Build history of the part. All positions in model axes, mm. A direction names the side the tool comes from. Give positions to 0.01 mm unless a question says otherwise; leave off trailing zeros. Loops run counter-clockwise (first coordinate to the right, second up) from the corner with the lowest first, then second, coordinate; pieces in that order, holes last. Notation, with made-up numbers: M 41.25,89.25 L 74.25,89.25 A16 ccw 74.25,106.25 Z; hole C 88.25,-24 d10. An arc over 180 degrees is marked long. Answer as a JSON object with one key per item and string values. Group by question number.
1. Slice it at C-C (z = -5). Give the number of separate pieces and of enclosed holes in the cut face, then the cut area to 3 significant figures.
2. Mould opens along Y. For faces 4 (the face through (9.203, 21.327, -2.555)), 5 (the face through (-0.03, 24.43, -56.15)), 6 (the face through (-6, 12, -2)) say: released by +Y, released by -Y, zero draft, split by the parting line, or undercut.
3. Drop flat-ended pins along their axis: pin 1 Ø5.5 at (x, z) = (0, -26.75) entering from +Y; pin 2 Ø6 at (y, z) = (3, -9.5) entering from +X; pin 3 Ø4 at (x, z) = (8.66, -5) entering from -Y; pin 4 Ø1.6 at (y, z) = (22.5, -49.5) entering from +X. Give the stop position or say it passes through.
4. 3-axis set-ups, long thin cutter, end or side, ignore diameter. For faces 1 (the face through (-1, 22.5, -25)), 2 (the face through (1, 19, -21.754)), 3 (the face through (-3, 2, -46)): which of +Z, -Z, +X, -X, +Y, -Y reach the whole face in a straight line?
5. Slice it at A-A (y = 19.25). List the corners of the cut face in (x, z) (3 decimals), then the cut area to 3 significant figures.
6. Slice it at B-B (y = 9.25). List the corners of the cut face in (x, z), then the cut area to 3 significant figures.
7. Drill centre lines: line 1 along Y through (x, z) = (11.75, -2.5); line 2 along Z through (x, y) = (-4.25, 11.75). Where is each one in solid material? Low to high. Write a range as [from, to].
from build123d import *

# Parameters (mm, degrees)
EXTRUDE_1_DEPTH           = 7.45
EXTRUDE_2_DEPTH           = 3.45
SKETCH_3_W                = 26
SKETCH_3_H                = 4
CUT_EXTRUDE_1_DEPTH       = 9.8
SKETCH_4_W                = 4.2
SKETCH_4_H                = 62.754310162
EXTRUDE_3_DEPTH           = 5.05
CUT_EXTRUDE_2_DEPTH       = 1.45
SKETCH_6_W                = 7.8
SKETCH_6_H                = 4
EXTRUDE_4_DEPTH           = 5.05
SKETCH_7_W                = 9.8
SKETCH_7_H                = 4
CUT_EXTRUDE_3_DEPTH       = 9
CUT_EXTRUDE_4_DEPTH       = 9.05
CUT_EXTRUDE_5_REACH       = 63.678
SKETCH_10_W               = 5.05
SKETCH_10_H               = 12
SKETCH_11_W               = 14
SKETCH_11_H               = 5.05
CUT_EXTRUDE_6_DEPTH       = 2.2
HOLE_WIZARD_1_D           = 5.01
HOLE_WIZARD_2_D           = 5.05
HOLE_WIZARD_3_D           = 5.05
HOLE_WIZARD_4_D           = 3.4
HOLE_WIZARD_4_DEPTH       = 12.5
HOLE_WIZARD_4_CBORE_D     = 6
HOLE_WIZARD_4_CBORE_DEPTH = 2.5
FILLET_1_R                = 5
FILLET_2_R                = 6
FILLET_3_R                = 0.5
FILLET_4_R                = 1
FILLET_5_R                = 2


# Read off the part's stored shape, not the designer's step: 镜向2
with BuildPart() as part:
    # 草图1 → 凸台-拉伸1 (new body)
    with BuildSketch(Plane(origin=(0, 7.45, 0), x_dir=(1, 0, 0), z_dir=(0, 1, 0))):
        with BuildLine():
            Line((6, 15.064661918), (6, 56.754310162))
            Line((6, 56.754310162), (-8, 56.754310162))
            Line((-8, 56.754310162), (-8, -6))
            Line((-8, -6), (1.607695155, -6))
            Line((1.607695155, -6), (11.660254038, -0.196152423))
            ThreePointArc((11.660254038, -0.196152423), (14.637422226, 4.477065544), (12.516979696, 9.596266659))
            Line((12.516979696, 9.596266659), (6, 15.064661918))
        make_face()
    extrude(amount=-EXTRUDE_1_DEPTH)

    # 草图2 → 凸台-拉伸2 (add)
    with BuildSketch(Plane.XZ):
        Polygon((6, -42.006832742), (6, -56.754310162), (7, -56.754310162), (7, -44.754310162), align=None)
    extrude(amount=-EXTRUDE_2_DEPTH)

    # 草图3 → 切除-拉伸1 (cut)
    with BuildSketch(Plane(origin=(6, 0, 0), x_dir=(0, 0, -1), z_dir=(1, 0, 0))):
        with Locations((43.754310162, 5.45)):
            Rectangle(SKETCH_3_W, SKETCH_3_H)
    extrude(amount=-CUT_EXTRUDE_1_DEPTH, mode=Mode.SUBTRACT)

    # 草图4 → 凸台-拉伸3 (add)
    with BuildSketch(Plane(origin=(0, 7.45, 0), x_dir=(-1, 0, 0), z_dir=(0, 1, 0))):
        with Locations((5.9, -25.377155081)):
            Rectangle(SKETCH_4_W, SKETCH_4_H)
    extrude(amount=EXTRUDE_3_DEPTH)

    # 草图5 → 切除-拉伸2 (cut)
    with BuildSketch(Plane(origin=(0, 3.45, 0), x_dir=(-1, 0, 0), z_dir=(0, 1, 0))):
        with BuildLine():
            Line((3.8, -30.754310162), (2.5, -30.754310162))
            Line((2.5, -30.754310162), (2.5, -46.9477369))
            ThreePointArc((2.5, -46.9477369), (2.258573906, -47.375684951), (1.76744186, -47.390361698))
            ThreePointArc((1.76744186, -47.390361698), (-3.252405192, -52.719471851), (3.8, -50.754310162))
            Line((3.8, -50.754310162), (3.8, -30.754310162))
        make_face()
    extrude(amount=-CUT_EXTRUDE_2_DEPTH, mode=Mode.SUBTRACT)

    # 草图6 → 凸台-拉伸4 (add)
    with BuildSketch(Plane(origin=(0, 7.45, 0), x_dir=(-1, 0, 0), z_dir=(0, 1, 0))):
        with Locations((-0.1, -10)):
            Rectangle(SKETCH_6_W, SKETCH_6_H)
    extrude(amount=EXTRUDE_4_DEPTH)

    # 草图7 → 切除-拉伸3 (cut)
    with BuildSketch(Plane(origin=(0, 0, -30.754310162), x_dir=(-1, 0, 0), z_dir=(0, 0, -1))):
        with Locations((-1.1, 5.45)):
            Rectangle(SKETCH_7_W, SKETCH_7_H)
    extrude(amount=-CUT_EXTRUDE_3_DEPTH, mode=Mode.SUBTRACT)

    # 草图8 → 切除-拉伸4 (cut)
    with BuildSketch(Plane(origin=(0, 12.5, 0), x_dir=(-1, 0, 0), z_dir=(0, 1, 0))):
        with BuildLine():
            Line((3.8, -45.792203754), (3.8, -55.716416569))
            ThreePointArc((3.8, -55.716416569), (6.25, -50.754310162), (3.8, -45.792203754))
        make_face()
    extrude(amount=-CUT_EXTRUDE_4_DEPTH, mode=Mode.SUBTRACT)

    # 草图10 → 切除-拉伸5 (cut, up to next)
    with BuildSketch(Plane(origin=(-6, 0, 0), x_dir=(0, -1, 0), z_dir=(-1, 0, 0)), mode=Mode.PRIVATE) as cut_extrude_5_sk1:
        with Locations((-9.975, -18)):
            Rectangle(SKETCH_10_W, SKETCH_10_H)
    cut_extrude_5_tool1 = extrude(cut_extrude_5_sk1.sketch, amount=-CUT_EXTRUDE_5_REACH, mode=Mode.PRIVATE) & part.part
    add(cut_extrude_5_tool1.solids().sort_by_distance((-6, 9.975, -18))[0], mode=Mode.SUBTRACT)

    # 草图11 → 切除-拉伸6 (cut)
    with BuildSketch(Plane(origin=(-3.8, 0, 0), x_dir=(0, 0, -1), z_dir=(1, 0, 0))):
        with Locations((1, 9.975)):
            Rectangle(SKETCH_11_W, SKETCH_11_H)
    extrude(amount=-CUT_EXTRUDE_6_DEPTH, mode=Mode.SUBTRACT)

    # 孔1 (through all)
    with Locations(Plane(origin=(0, 7.45, 0), x_dir=(1, 0, 0), z_dir=(0, 1, 0))):
        with Locations((8.660254038, 5)):
            Hole(HOLE_WIZARD_1_D / 2)

    # 孔2 (through all)
    with Locations(Plane(origin=(0, 7.45, 0), x_dir=(1, 0, 0), z_dir=(0, 1, 0))):
        with Locations((0, 0)):
            Hole(HOLE_WIZARD_2_D / 2)

    # 孔3 (through all)
    with Locations(Plane(origin=(0, 2, 0), x_dir=(1, 0, 0), z_dir=(0, 1, 0))):
        with Locations((0, 50.754310162)):
            Hole(HOLE_WIZARD_3_D / 2)

    # 孔4
    with Locations(Plane(origin=(0, 0, 0), x_dir=(-1, 0, 0), z_dir=(0, -1, 0))):
        with Locations((0, 26.754310162)):
            CounterBoreHole(HOLE_WIZARD_4_D / 2, HOLE_WIZARD_4_CBORE_D / 2, HOLE_WIZARD_4_CBORE_DEPTH, depth=HOLE_WIZARD_4_DEPTH)

    # 圆角1
    fillet_1_edges = [part.edges().sort_by_distance(p)[0] for p in [
        (6, 3.725, -15.064661918),
        (6, 1.725, -42.006832742),
        (7, 1.725, -56.754310162),
    ]]
    fillet(fillet_1_edges, radius=FILLET_1_R)

    # 圆角2
    fillet_2_edges = [part.edges().sort_by_distance(p)[0] for p in [
        (-8, 6.25, -56.754310162),
        (-8, 6.25, 6),
        (1.607695155, 3.725, 6),
    ]]
    fillet(fillet_2_edges, radius=FILLET_2_R)

    # 圆角3
    fillet_3_edges = [part.edges().sort_by_distance(p)[0] for p in [
        (-2.5, 2.725, -30.754310162),
        (-3.8, 2.725, -30.754310162),
    ]]
    fillet(fillet_3_edges, radius=FILLET_3_R)

    # 圆角4
    fillet_4_edges = [part.edges().sort_by_distance(p)[0] for p in [
        (-4.9, 7.45, -24),
        (-1, 7.45, -8),
        (-1, 7.45, -12),
        (1.1, 3.45, -21.754310162),
    ]]
    fillet(fillet_4_edges, radius=FILLET_4_R)

    # 圆角5
    fillet_5_edges = [part.edges().sort_by_distance(p)[0] for p in [
        (6, 0, -29.260699024),
        (0, 0, -56.754310162),
        (7, 0, -48.254310162),
        (5.535533906, 0, -55.289844068),
        (6.075961235, 0, -41.993438727),
        (6.468461065, 0, -15.2831089),
        (-8, 0, -25.377155081),
        (7.330127019, 0, 2.696152423),
        (-1, 0, 6),
        (1.552914271, 0, 5.795554958),
        (-6.242640687, 0, 4.242640687),
        (-6.242640687, 0, -54.996950849),
        (6.650768448, 0, -43.794804359),
        (14.637422226, 0, -4.477065544),
        (10.151520824, 0, -11.581122326),
    ]]
    fillet(fillet_5_edges, radius=FILLET_5_R)

    # 镜向2: part across plane


with BuildPart() as part_1:
    add(part.part)
    add(part.part.mirror(Plane.ZX.offset(12.5)))


solid = part_1.part
Established:
{
 "1": {"separate pieces": "3", "enclosed holes": "0", "area": "280 mm^2"},
 "2": {"face 4": "zero draft", "face 5": "released by +Y", "face 6": "undercut"},
 "3": {"pin 1": "stops at y = 22.5", "pin 2": "stops at x = 14.47", "pin 3": "passes through", "pin 4": "stops at x = 7"},
 "4": {"face 1": "+Y", "face 2": "-Z, +X", "face 3": "none"},
 "5": {"outline": "M -8,-50.754 A6 ccw -3.8,-56.478 L -3.8,-55.716 A6.25 cw -3.8,-45.792 L -3.8,-21.754 L 6,-21.754 L 6,-17.396 A5 cw 7.786,-13.566 L 12.517,-9.596 A6 ccw 11.66,0.196 L 3,5.196 A6 ccw 0,6 L -2,6 A6 ccw -8,0 Z; hole C 0,0 d5.05; hole C 8.66,-5 d5.01", "area": "563 mm^2"},
 "6": {"outline": "M -8,-50.75 A6 ccw -3.8,-56.48 L -3.8,-55.72 A6.25 cw -3.8,-45.79 L -3.8,-24 L -6,-24 L -6,-12 L 4,-12 L 4,-8 L -6,-8 L -6,4.47 A6 ccw -8,0 Z", "area": "207 mm^2"},
 "7": {"line 1": "y = [0, 7.45], [17.55, 25]", "line 2": "z = [-56.32, -55.34], [-46.17, -24], [-12, -8]"}
}
